Could you check a few things on this model? Use its own coordinates, in mm. Give positions to 0.01 mm unless a question says otherwise; leave off trailing zeros. Loops run counter-clockwise (first coordinate to the right, second up) from the corner with the lowest first, then second, coordinate; pieces in that order, holes last.
1. I need wall thicknesses on line 1 along Y through (x, z) = (0, 23.5); line 2 along Z through (x, y) = (-0.5, 33) (3 decimals); line 3 along Z through (x, y) = (7, 31.5). Which ranges of each line are inside material? Lowest first, please.
2. Imagine slicing it at B-B (x = 0). List the corners of the cut face in (y, z) for me, plus the area to 3 significant figures.
3. Imagine slicing it at A-A (z = 0). List the corners of the cut face in (x, y) for me, plus the area to 3 significant figures.
4. Thinking about a two-plate mould opening in Y: for faces 1 (the cylindrical face through (-0.54, 47.44, -23.41)), 2 (the flat face through (-22.1, 60, 1.7)), 3 (the flat face through (-22.1, 0, 1.7)), which applies, +Y half, -Y half, draft (parallel to the pull), parting line (faces both ways), or undercut?
5. For P1, Ø3, axis at x = 12, y = 33.5, coming from the +Z side; P2, Ø1, axis at x = 10.5, y = 39.5, coming from the -Z side; P3, Ø4, axis at x = 0, y = 45, coming from the -Z side; P4, Ø1.5, axis at x = 10.5, y = 54, coming from the -Z side, each with a flat end and sliding along its axis, tell me the tip position at first contact or that it passes through.
```python
from build123d import *

# Parameters (mm, degrees)
ESBO_O1_R                = 25
ESBO_O1_R_2              = 22
RESSALTO_EXTRUS_O1_DEPTH = 60
ESBO_O2_R                = 2.5
CORTE_EXTRUS_O1_DEPTH    = 70.641941386


with BuildPart() as part:
    # Esboço1 → Ressalto-extrusão1 (new body)
    with BuildSketch(Plane(origin=(0, 0, 0), x_dir=(1, 0, 0), z_dir=(0, 1, 0))):
        with Locations(Location((0, 0, 0), (0, 0, 270))):
            Circle(ESBO_O1_R)
        with Locations(Location((0, 0, 0), (0, 0, 270))):
            Circle(ESBO_O1_R_2, mode=Mode.SUBTRACT)
    extrude(amount=RESSALTO_EXTRUS_O1_DEPTH)

    # Esboço2 → Corte-extrusão1 (cut, symmetric)
    with BuildSketch(Plane.XY):
        with Locations((0, 15)):
            Circle(ESBO_O2_R)
    corte_extrus_o1 = extrude(amount=CORTE_EXTRUS_O1_DEPTH, both=True, mode=Mode.SUBTRACT)

    # Espelhar1: Corte-extrusão1 across plane
    add(corte_extrus_o1.mirror(Plane(origin=(0, 30, 0), x_dir=(0, 0, 1), z_dir=(0, -1, 0))), mode=Mode.SUBTRACT)


solid = part.part
```
Derived:
1. line 1: y = 0 to 12.5, 17.5 to 42.5, 47.5 to 60
1. line 2: z = -24.995 to -21.994, 21.994 to 24.995
1. line 3: z = -24 to -20.86, 20.86 to 24
2. outline: (0, -25) - (12.5, -25) - (12.5, -22) - (0, -22) - close; (0, 22) - (12.5, 22) - (12.5, 25) - (0, 25) - close; (17.5, -25) - (42.5, -25) - (42.5, -22) - (17.5, -22) - close; (17.5, 22) - (42.5, 22) - (42.5, 25) - (17.5, 25) - close; (47.5, -25) - (60, -25) - (60, -22) - (47.5, -22) - close; (47.5, 22) - (60, 22) - (60, 25) - (47.5, 25) - close
2. area: 300 mm2
3. outline: (-25, 0) - (-22, 0) - (-22, 60) - (-25, 60) - close; (22, 0) - (25, 0) - (25, 60) - (22, 60) - close
3. area: 360 mm2
4. face 1: undercut
4. face 2: +Y half
4. face 3: -Y half
5. P1: stops at z = 22.69
5. P2: stops at z = -22.91
5. P3: passes through
5. P4: stops at z = -23.02
